from build123d import *

# Parameters (mm, degrees)
SKETCH1_W           = 41.6
SKETCH1_H           = 20
SKETCH1_W_2         = 39.6
SKETCH1_H_2         = 18
BOSS_EXTRUDE2_DEPTH = 10
SKETCH2_W           = 4
SKETCH2_H           = 10
BOSS_EXTRUDE3_DEPTH = 1
SKETCH3_W           = 3
SKETCH3_H           = 1
CUT_EXTRUDE1_DEPTH  = 27
SKETCH4_W           = 4
SKETCH4_H           = 10
BOSS_EXTRUDE4_DEPTH = 1
SKETCH5_W           = 3
SKETCH5_H           = 1
CUT_EXTRUDE2_DEPTH  = 27
SKETCH6_W           = 41.6
SKETCH6_H           = 20
SKETCH6_W_2         = 39.6
SKETCH6_H_2         = 18
BOSS_EXTRUDE6_DEPTH = 19
SKETCH7_W           = 41.6
SKETCH7_H           = 20
BOSS_EXTRUDE7_DEPTH = 1


with BuildPart() as part:
    # Sketch1 → Boss-Extrude2 (new body)
    with BuildSketch(Plane.XY):
        Rectangle(SKETCH1_W, SKETCH1_H)
        Rectangle(SKETCH1_W_2, SKETCH1_H_2, mode=Mode.SUBTRACT)
    extrude(amount=BOSS_EXTRUDE2_DEPTH)

    # Sketch2 → Boss-Extrude3 (add)
    with BuildSketch(Plane.XZ.offset(10)):
        with Locations((-11.3, 5)):
            Rectangle(SKETCH2_W, SKETCH2_H)
        with Locations((11.3, 5)):
            Rectangle(SKETCH2_W, SKETCH2_H)
    extrude(amount=BOSS_EXTRUDE3_DEPTH)

    # Sketch3 → Cut-Extrude1 (cut)
    with BuildSketch(Plane.ZY.offset(13.3)):
        Polygon((8.900149248, -10), (7, -11), (10, -11), (10, -10), align=None)
        with Locations((1.5, -10.5)):
            Rectangle(SKETCH3_W, SKETCH3_H)
    extrude(amount=-CUT_EXTRUDE1_DEPTH, mode=Mode.SUBTRACT)

    # Sketch4 → Boss-Extrude4 (add)
    with BuildSketch(Plane(origin=(0, 10, 0), x_dir=(1, 0, 0), z_dir=(0, 1, 0))):
        with Locations((11.3, -5)):
            Rectangle(SKETCH4_W, SKETCH4_H)
        with Locations((-11.3, -5)):
            Rectangle(SKETCH4_W, SKETCH4_H)
    extrude(amount=BOSS_EXTRUDE4_DEPTH)

    # Sketch5 → Cut-Extrude2 (cut)
    with BuildSketch(Plane(origin=(13.3, 0, 0), x_dir=(0, 0, -1), z_dir=(1, 0, 0))):
        Polygon((-7, 11), (-10, 11), (-10, 10), (-8.900149248, 10), align=None)
        with Locations((-1.5, 10.5)):
            Rectangle(SKETCH5_W, SKETCH5_H)
    extrude(amount=-CUT_EXTRUDE2_DEPTH, mode=Mode.SUBTRACT)

    # Sketch6 → Boss-Extrude6 (add)
    with BuildSketch(Plane(origin=(0, 0, 0), x_dir=(-1, 0, 0), z_dir=(0, 0, -1))):
        Rectangle(SKETCH6_W, SKETCH6_H)
        Rectangle(SKETCH6_W_2, SKETCH6_H_2, mode=Mode.SUBTRACT)
    extrude(amount=BOSS_EXTRUDE6_DEPTH)

    # Sketch7 → Boss-Extrude7 (add)
    with BuildSketch(Plane(origin=(0, 0, -19), x_dir=(-1, 0, 0), z_dir=(0, 0, -1))):
        Rectangle(SKETCH7_W, SKETCH7_H)
    extrude(amount=BOSS_EXTRUDE7_DEPTH)


solid = part.part
Design review of the part built by this model. Coordinates are the model's own, in mm. A direction names the side the tool comes from. Coordinates: 2 decimals unless noted, no trailing zeros. Order: outer loops, then holes, each group sorted by start corner. A loop starts at its lowest first (then second) coordinate and runs counter-clockwise, first axis right, second up. Notation, with made-up numbers: M -26.75,78.25 L -19.75,78.25 A21 ccw -19.75,84.25 Z; hole C 76.5,29 d1. An arc over 180 degrees is marked long. Use a Markdown table: item, result.
(1) For P1, Ø4, axis at x = -7.5, z = -14, coming from the +Y side; P2, Ø1.1, axis at y = -10.5, z = 7, coming from the +X side; P3, Ø4, axis at x = -5.5, y = 4.5, coming from the +Z side; P4, Ø0.8, axis at x = 11, y = 10.5, coming from the -Z side, all flat-tipped, find the tip position at first contact; note any pin that passes through.
Worked answers:
| item | result |
|---|---|
| P1 | stops at y = 10 |
| P2 | stops at x = 20.8 |
| P3 | stops at z = -19 |
| P4 | stops at z = 3 |
(2) Draft analysis for pull direction Y (two halves, no side actions). For faces 1 (the flat face through (-11, -11, 5)), 2 (the flat face through (0, 0, -19)), 3 (the flat face through (13.3, -10.5, 5.3)), state which applies: released by +Y, released by -Y, zero draft, split by the parting line, or undercut.
Worked answers:
| item | result |
|---|---|
| face 1 | released by -Y |
| face 2 | undercut |
| face 3 | zero draft |
(3) Add section A-A (y = 2.5). Give the boundary of the cut face in (x, z).
Worked answers:
| item | result |
|---|---|
| outline | M -20.8,-20 L 20.8,-20 L 20.8,10 L 19.8,10 L 19.8,-19 L -19.8,-19 L -19.8,10 L -20.8,10 Z |
(4) Add section C-C (x = -18). Give the boundary of the cut face in (y, z), then the cut area to 3 significant figures.
Worked answers:
| item | result |
|---|---|
| outline | M -10,-20 L 10,-20 L 10,10 L 9,10 L 9,-19 L -9,-19 L -9,10 L -10,10 Z |
| area | 78.0 mm2 |
(5) Add section B-B (z = -15). Give the boundary of the cut face in (x, y).
Worked answers:
| item | result |
|---|---|
| outline | M -20.8,-10 L 20.8,-10 L 20.8,10 L -20.8,10 Z; hole M -19.8,-9 L 19.8,-9 L 19.8,9 L -19.8,9 Z |
(6) Add section D-D (x = 12.5). Give the boundary of the cut face in (y, z).
Worked answers:
| item | result |
|---|---|
| outline | M -11,3 L -10,3 L -10,-20 L 10,-20 L 10,3 L 11,3 L 11,7 L 10,8.9 L 10,10 L 9,10 L 9,-19 L -9,-19 L -9,10 L -10,10 L -10,8.9 L -11,7 Z |
(7) For faces 4 (the flat face through (19.8, 0, -4)), 5 (the flat face through (11.3, 10.5, 3)), 6 (the flat face through (13.3, 10.5, 5.3)), 7 (the flat face through (-9.3, 10.5, 5.3)), 8 (the flat face through (-13.3, 10.5, 5.3)), list the 3-axis set-ups (+Z, -Z, +X, -X, +Y, -Y) from which the entire face can be reached by the end or side of a thin tool; tool diameter is ignored.
Worked answers:
| item | result |
|---|---|
| face 4 | +Z |
| face 5 | -Z, +X, -X, +Y |
| face 6 | +Z, -Z, +X, +Y |
| face 7 | +Z, -Z, +Y |
| face 8 | +Z, -Z, -X, +Y |
(8) Wall thickness on probe 1 along Y at (x, z) = (18.5, -2.5); probe 2 along X at (y, z) = (-3, 7.75); probe 3 along Z at (x, y) = (4, 0.75): over which ranges is each line inside the solid? List them lowest first.
Worked answers:
| item | result |
|---|---|
| probe 1 | y = -10 to -9, 9 to 10 |
| probe 2 | x = -20.8 to -19.8, 19.8 to 20.8 |
| probe 3 | z = -20 to -19 |
